```python
from build123d import *

# Parameters (mm, degrees)
BOSS_EXTRUDE1_DEPTH      = 101.6
CUT_EXTRUDE1_START       = -2.54
CUT_EXTRUDE1_DEPTH       = 2.54
BOSS_EXTRUDE2_DEPTH      = 2.54
CHAMFER2_SIZE            = 2.54
BOSS_EXTRUDE5_DEPTH      = 2.54
CHAMFER2_OF_MIRROR1_SIZE = 2.54
MIRROR3_COPY_1_DEPTH     = 2.54
MIRROR3_COPY_2_DEPTH     = 2.54
LPATTERN14_COUNT         = 10
LPATTERN14_PITCH         = 180.086
CHAMFER3_SIZE            = 2.54
CHAMFER4_SIZE            = 2.54


with BuildPart() as part:
    # Sketch1 → Boss-Extrude1 (new body)
    with BuildSketch(Plane(origin=(0, 0, 0), x_dir=(1, 0, 0), z_dir=(0, 1, 0))):
        with BuildLine():
            Line((63.390989336, 0), (90.060989336, 0))
            Line((90.060989336, 0), (90.060989336, 95.25))
            Line((90.060989336, 95.25), (-90.060989336, 95.25))
            Line((-90.060989336, 95.25), (-90.060989336, 0))
            Line((-90.060989336, 0), (-63.390989336, 0))
            ThreePointArc((-63.390989336, 0), (0, 59.780796989), (63.390989336, 0))
        make_face()
    boss_extrude1 = extrude(amount=BOSS_EXTRUDE1_DEPTH)

    # Sketch2 → Cut-Extrude1 (cut)
    with BuildSketch(Plane(origin=(0, 101.6, 0), x_dir=(1, 0, 0), z_dir=(0, 1, 0)).offset(CUT_EXTRUDE1_START)):
        with BuildLine():
            Line((67.194448696, 0.223152181), (63.390989336, 0))
            ThreePointArc((63.390989336, 0), (0, 59.780796989), (-63.390989336, 0))
            Line((-63.390989336, 0), (-67.194448696, 0.223152181))
            ThreePointArc((-67.194448696, 0.223152181), (0, 63.590796989), (67.194448696, 0.223152181))
        make_face()
    cut_extrude1 = extrude(amount=CUT_EXTRUDE1_DEPTH, mode=Mode.SUBTRACT)

    # Sketch3 → Boss-Extrude2 (add)
    with BuildSketch(Plane(origin=(0, 101.6, 0), x_dir=(1, 0, 0), z_dir=(0, 1, 0))):
        with BuildLine():
            Line((-70.997908056, 0.446304361), (-67.194448696, 0.223152181))
            ThreePointArc((-67.194448696, 0.223152181), (0, 63.590796989), (67.194448696, 0.223152181))
            Line((67.194448696, 0.223152181), (70.997908056, 0.446304361))
            ThreePointArc((70.997908056, 0.446304361), (0, 67.400796989), (-70.997908056, 0.446304361))
        make_face()
    boss_extrude2 = extrude(amount=BOSS_EXTRUDE2_DEPTH)

    # Chamfer2
    chamfer2_edges = [part.edges().sort_by_distance(p)[0] for p in [
        (0, 99.06, -59.780796989),
    ]]
    chamfer(chamfer2_edges, length=CHAMFER2_SIZE)

    # Sketch4 → Boss-Extrude5 (add)
    with BuildSketch(Plane.XY):
        with BuildLine():
            Line((-90.060989336, 50.8), (-63.390989336, 50.8))
            Line((-63.390989336, 50.8), (-63.390989336, 104.14))
            ThreePointArc((-63.390989336, 104.14), (-71.202451482, 122.998537854), (-90.060989336, 130.81))
            Line((-90.060989336, 130.81), (-90.060989336, 50.8))
        make_face()
    boss_extrude5 = extrude(amount=BOSS_EXTRUDE5_DEPTH)

    # Mirror1: Cut-Extrude1, Boss-Extrude2, Boss-Extrude5 across plane
    add(cut_extrude1.mirror(Plane.ZX.offset(50.8)), mode=Mode.SUBTRACT)
    add(boss_extrude2.mirror(Plane.ZX.offset(50.8)))
    add(boss_extrude5.mirror(Plane.ZX.offset(50.8)))

    # Chamfer2 of Mirror1
    chamfer2_of_mirror1_edges = [part.edges().sort_by_distance(p)[0] for p in [
        (0, 2.54, -59.780796989),
    ]]
    chamfer(chamfer2_of_mirror1_edges, length=CHAMFER2_OF_MIRROR1_SIZE)

    # Mirror2: Boss-Extrude5 across plane
    add(boss_extrude5.mirror(Plane(origin=(0, 0, 0), x_dir=(0, 0, 1), z_dir=(1, 0, 0))))

    # Mirror3 copy 1 sketch → Mirror3 copy 1 (add)
    with BuildSketch(Plane(origin=(0, 101.6, 0), x_dir=(-1, 0, 0), z_dir=(0, 0, 1))):
        with BuildLine():
            Line((-90.060989336, 50.8), (-63.390989336, 50.8))
            Line((-63.390989336, 50.8), (-63.390989336, 104.14))
            ThreePointArc((-63.390989336, 104.14), (-71.202451482, 122.998537854), (-90.060989336, 130.81))
            Line((-90.060989336, 130.81), (-90.060989336, 50.8))
        make_face()
    extrude(amount=MIRROR3_COPY_1_DEPTH)

    # Mirror3 copy 2 sketch → Mirror3 copy 2 (add)
    with BuildSketch(Plane(origin=(0, 101.6, 0), x_dir=(1, 0, 0), z_dir=(0, 0, 1))):
        with BuildLine():
            Line((-90.060989336, -50.8), (-63.390989336, -50.8))
            Line((-63.390989336, -50.8), (-63.390989336, -104.14))
            ThreePointArc((-63.390989336, -104.14), (-71.202451482, -122.998537854), (-90.060989336, -130.81))
            Line((-90.060989336, -130.81), (-90.060989336, -50.8))
        make_face()
    extrude(amount=MIRROR3_COPY_2_DEPTH)

    # LPattern14: Boss-Extrude1, Cut-Extrude1, Boss-Extrude2 ×10
    with Locations(*[(-i * LPATTERN14_PITCH, 0, 0) for i in range(1, LPATTERN14_COUNT)]):
        add(boss_extrude1)
        add(cut_extrude1, mode=Mode.SUBTRACT)
        add(boss_extrude2)

    # Chamfer3
    chamfer3_edges = [part.edges().sort_by_distance(p)[0] for p in [
        (-810.387, 101.6, -95.25),
    ]]
    chamfer(chamfer3_edges, length=CHAMFER3_SIZE)

    # Chamfer4
    chamfer4_edges = [part.edges().sort_by_distance(p)[0] for p in [
        (90.060989336, 50.8, 2.54),
        (-1710.834989336, 50.8, 0),
        (90.060989336, 49.53, -95.25),
        (-810.387, 0, -95.25),
    ]]
    chamfer(chamfer4_edges, length=CHAMFER4_SIZE)


solid = part.part
```
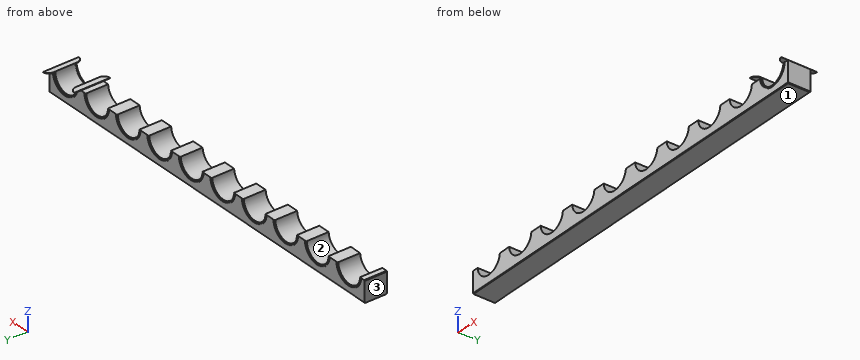
Check sheet for the modelled part. Datum: model origin and axes. Units: mm. Face numbers are marked on the shaded views. Round coordinates to 2 decimals unless told otherwise and drop trailing zeros. Loops run counter-clockwise (first coordinate to the right, second up) from the corner with the lowest first, then second, coordinate; pieces in that order, holes last. Notation, with made-up numbers: (-28.5, 42) - (1.5, 42) arc R31 ccw to (1.5, 75) - close; hole circle Ø9 at (-37.75, 83.5). An arc over 180 degrees is marked (long way). Answer as a JSON object with one key per item and string values. Group by question number.
Q1. Sectioned sample at C-C, the plane z = -24. Count the separate pieces of the cut face and the enclosed holes in it, plus the area to 3 significant figures.
Q2. Mould release check, pull along X, two halves, no side actions. Record for the marked faces 1, 2 and 3: released by +X, released by -X, zero draft, split by the parting line, or undercut.
Q3. Sectioned sample at A-A, the plane x = -900.43. Enter the section's corners in (y, z), plus the area to 3 significant figures.
Q4. Gauge pin test, flat ends, axial feed: P1, Ø4, axis at x = -797, z = -47, coming from the +Y side; P2, Ø16, axis at x = -1169, y = 66.5, coming from the +Z side; P3, Ø8, axis at x = 74.5, y = 123.5, coming from the -Z side. Record the tip position at first contact, or that the pin passes through.
Q5. Scan lines: line 1 along Y through (x, z) = (-778, -87.5); line 2 along Y through (x, z) = (-1196, -17.5); line 3 along Z through (x, y) = (-266.5, 49.5). Record each from-to range of solid material in increasing order. Write a range as [from, to].
Q6. Sectioned sample at D-D, the plane x = 0. Enter the section's corners in (y, z), plus the area to 3 significant figures.
Solution:
{
 "1": {"separate pieces": "11", "enclosed holes": "0", "area": "66,900 mm²"},
 "2": {"face 1": "zero draft", "face 2": "undercut", "face 3": "released by -X"},
 "3": {"outline": "(0, -92.71) - (2.54, -95.25) - (99.06, -95.25) - (101.6, -92.71) - (101.6, -67.4) - (104.14, -67.4) - (104.14, -63.59) - (99.06, -63.59) - (99.06, -59.78) - (0, -59.78) - close", "area": "3,600 mm²"},
 "4": {"P1": "stops at y = 101.6", "P2": "stops at z = 0", "P3": "stops at z = 0"},
 "5": {"line 1": "y = [0, 101.6]", "line 2": "y = [0, 104.14]", "line 3": "z = [-95.25, 0]"},
 "6": {"outline": "(-2.54, -67.4) - (0, -67.4) - (0, -92.71) - (2.54, -95.25) - (99.06, -95.25) - (101.6, -92.71) - (101.6, -67.4) - (104.14, -67.4) - (104.14, -63.59) - (99.06, -63.59) - (99.06, -62.32) - (96.52, -59.78) - (5.08, -59.78) - (2.54, -62.32) - (2.54, -63.59) - (-2.54, -63.59) - close", "area": "3,590 mm²"}
}
